Input: dimensioned drawing with shaded views. Units: mm. Origin: part minimum x, y, z. A direction names the side the tool comes from. Round coordinates to 2 decimals unless told otherwise and drop trailing zeros. Order: outer loops, then holes, each group sorted by start corner. A loop starts at its lowest first (then second) coordinate and runs counter-clockwise, first axis right, second up. Notation, with made-up numbers: M 50.25,-7.75 L 75.25,-7.75 A10 cw 75.25,6.25 Z; hole C 81,32 d6. An arc over 180 degrees is marked long. Answer as CSV lines item,"result". Start each with the question number.
Item 1: Section query B-B on z = 40. Return the cut outline in (x, y).
Item 2: Section query C-C on y = 79. Return the cut outline in (x, z).
Item 3: Line query: line 1 (Y direction, x = 95, z = 48.5); line 2 (X direction, y = 141, z = 56.5); line 3 (Z direction, x = 190, y = 170). Output: solid intervals per line, ascending. Write a range as [from, to].
Item 4: Pull-direction query (Y, two-part tool) for the marked faces 3, 4, 5 and 6; classes: +Y half, -Y half, draft (parallel to the pull), parting line (faces both ways), or undercut.
Item 5: Set-up query: the marked faces 1 and 2. Return all of +Z, -Z, +X, -X, +Y, -Y with unobstructed straight access to the full face (end or side cutting, diameter ignored); none if empty.
Item 6: Section query A-A on z = 65. Return the cut outline in (x, y), plus the area to 3 significant figures.
Item 7: First-contact query: P1, Ø6, axis at x = 86.5, z = 17.5, coming from the -Y side; P2, Ø10, axis at x = 327.5, y = 156, coming from the +Z side. Flat tips, straight axial feed; report the tip coordinate or a pass-through.
Item 8: Section query D-D on x = 287.5. Return the cut outline in (y, z), plus the area to 3 significant figures.
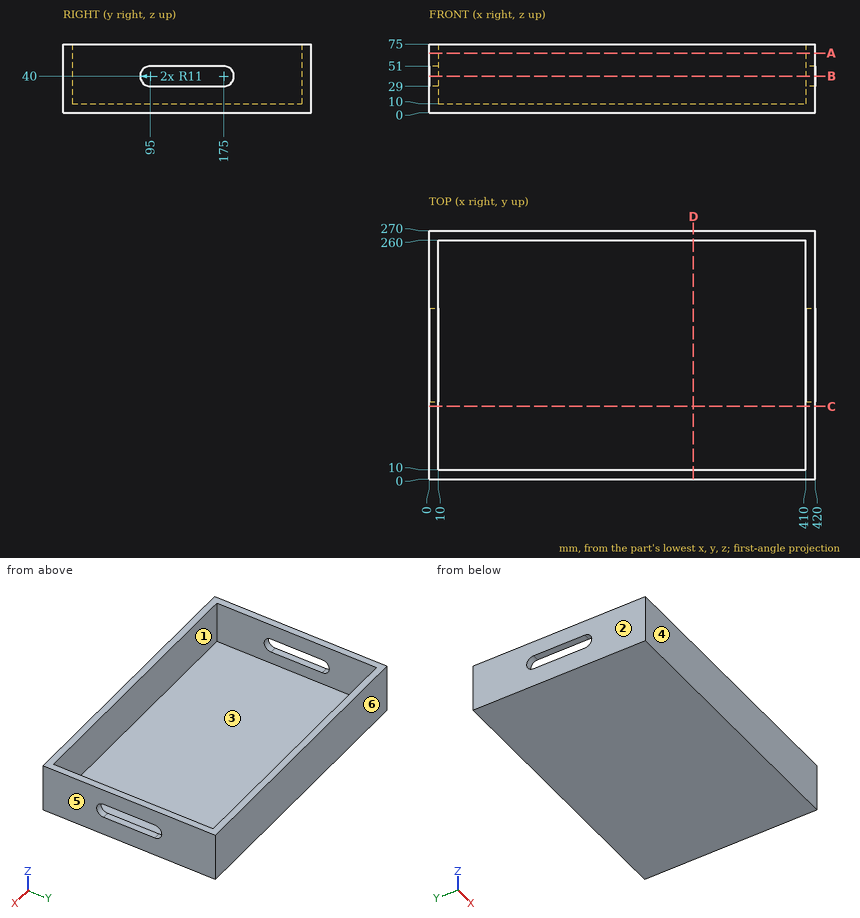
Results:
1,outline,"M 0,0 L 420,0 L 420,84 L 410,84 L 410,10 L 10,10 L 10,84 L 0,84 Z; M 0,186 L 10,186 L 10,260 L 410,260 L 410,186 L 420,186 L 420,270 L 0,270 Z"
2,outline,"M 0,0 L 420,0 L 420,75 L 410,75 L 410,10 L 10,10 L 10,75 L 0,75 Z"
3,line 1,"[0, 10], [260, 270]"
3,line 2,"[0, 10], [410, 420]"
3,line 3,"[0, 10]"
4,face 3,"undercut"
4,face 4,"-Y half"
4,face 5,"draft"
4,face 6,"+Y half"
5,face 1,"+Z"
5,face 2,"+Z, -Z, -X, +Y, -Y"
6,outline,"M 0,0 L 420,0 L 420,270 L 0,270 Z; hole M 10,10 L 410,10 L 410,260 L 10,260 Z"
6,area,"13,400 mm^2"
7,P1,"y = 0"
7,P2,"z = 10"
8,outline,"M 0,0 L 270,0 L 270,75 L 260,75 L 260,10 L 10,10 L 10,75 L 0,75 Z"
8,area,"4,000 mm^2"
